```python
from build123d import *

# Parameters (mm, degrees)
BOSS_EXTRUDE1_DEPTH  = 3.175
M5_CLEARANCE_HOLE1_D = 5.5


with BuildPart() as part:
    # Sketch1 → Boss-Extrude1 (new body)
    with BuildSketch(Plane(origin=(0, 0, 0), x_dir=(1, 0, 0), z_dir=(0, 1, 0))):
        Polygon((101.6, 0), (101.6, 69.088), (3.175, 69.088), (3.175, 57.15), (0, 57.15), (0, 44.45), (3.175, 44.45), (3.175, 31.75), (0, 31.75), (0, 19.05), (3.175, 19.05), (3.175, 0), align=None)
        Polygon((200.025, 69.088), (101.6, 69.088), (101.6, 0), (200.025, 0), (200.025, 19.05), (203.2, 19.05), (203.2, 31.75), (200.025, 31.75), (200.025, 44.45), (203.2, 44.45), (203.2, 57.15), (200.025, 57.15), align=None)
    extrude(amount=BOSS_EXTRUDE1_DEPTH)

    # M5 Clearance Hole1 (through all)
    with Locations(Plane(origin=(0, 3.175, 0), x_dir=(1, 0, 0), z_dir=(0, 1, 0))):
        with Locations((15.875, 61.468), (187.325, 61.468)):
            Hole(M5_CLEARANCE_HOLE1_D / 2)


solid = part.part
```
Geometry: final body of the model. Coordinates: model frame, mm. Coordinates: 2 decimals unless noted, no trailing zeros. Order: outer loops, then holes, each group sorted by start corner. A loop starts at its lowest first (then second) coordinate and runs counter-clockwise, first axis right, second up. Notation, with made-up numbers: M 77.25,0.5 L 128.25,0.5 A24 ccw 128.25,36.5 Z; hole C 76.5,-20 d4. An arc over 180 degrees is marked long. Answer in a Markdown table with one row per item. Add a question column.
Q1. Mould query, pull axis X, two halves, no side actions, for faces 1 (the cylindrical face through (190.072, 1.565, -61.589)), 2 (the flat face through (100, 3.175, -35)). Classes: released by +X, released by -X, zero draft, split by the parting line, or undercut.
Q2. Section query A-A on x = 187. Return the cut outline in (y, z) (3 decimals), and give its area (3 significant figures).
Q3. Contact query for flat-ended pins moving along their axis: P1, Ø1.6, axis at y = 2, z = -12, coming from the -X side (3 decimals); P2, Ø1, axis at x = 201.5, y = 1, coming from the -Z side; P3, Ø1, axis at x = 202, y = 2, coming from the +Z side. Output: stop coordinate, or through.
Q4. Section query B-B on y = 1.85. Return the cut outline in (x, z) (3 decimals), and give its area (3 significant figures).
Q5. Section query C-C on z = -39. Return the cut outline in (x, y) (3 decimals).
Q6. Line query: L1, parallel to X at y = 0.3, z = -61.5 (3 decimals); L2, parallel to X at y = 1.85, z = -15.5 (3 decimals). Output: solid intervals per line, ascending.
Completed:
| question | item | result |
|---|---|---|
| 1 | face 1 | undercut |
| 1 | face 2 | zero draft |
| 2 | outline | M 0,-69.088 L 3.175,-69.088 L 3.175,-64.199 L 0,-64.199 Z; M 0,-58.737 L 3.175,-58.737 L 3.175,0 L 0,0 Z |
| 2 | area | 202 mm2 |
| 3 | P1 | stops at x = 3.175 |
| 3 | P2 | stops at z = -57.15 |
| 3 | P3 | stops at z = -19.05 |
| 4 | outline | M 0,-57.15 L 3.175,-57.15 L 3.175,-69.088 L 200.025,-69.088 L 200.025,-57.15 L 203.2,-57.15 L 203.2,-44.45 L 200.025,-44.45 L 200.025,-31.75 L 203.2,-31.75 L 203.2,-19.05 L 200.025,-19.05 L 200.025,0 L 3.175,0 L 3.175,-19.05 L 0,-19.05 L 0,-31.75 L 3.175,-31.75 L 3.175,-44.45 L 0,-44.45 Z; hole C 15.875,-61.468 d5.5; hole C 187.325,-61.468 d5.5 |
| 4 | area | 13,700 mm2 |
| 5 | outline | M 3.175,0 L 200.025,0 L 200.025,3.175 L 3.175,3.175 Z |
| 6 | L1 | x = 3.175 to 13.125, 18.625 to 184.575, 190.075 to 200.025 |
| 6 | L2 | x = 3.175 to 200.025 |
